from build123d import *

# Parameters (mm, degrees)
F0_W     = 31
F0_H     = 13
F1_DEPTH = 2
F2_R     = 1.55
F3_DEPTH = 25
F4_R     = 2
F5_W     = 15
F5_H     = 5
F6_DEPTH = 25
F7_R     = 1
F8_R     = 0.2


with BuildPart() as f1:
    # F0 (on Front) → F1 (new body)
    with BuildSketch(Plane.XZ):
        with Locations((15.5, 6.5)):
            Rectangle(F0_W, F0_H)
    extrude(amount=F1_DEPTH)

    # F2 (on face) → F3 (cut)
    with BuildSketch(Plane.XZ.offset(2)):
        with Locations((4, 10)):
            Circle(F2_R)
        with Locations((4, 3)):
            Circle(F2_R)
        with Locations((27, 10)):
            Circle(F2_R)
        with Locations((27, 3)):
            Circle(F2_R)
    extrude(amount=-F3_DEPTH, mode=Mode.SUBTRACT)

    # F4
    f4_edges = [f1.edges().sort_by_distance(p)[0] for p in [
        (31, -1, 13),
        (31, -1, 0),
        (0, -1, 0),
        (0, -1, 13),
    ]]
    fillet(f4_edges, radius=F4_R)

    # F5 (on face) → F6 (cut)
    with BuildSketch(Plane.XZ.offset(2)):
        with Locations((15.5, 6.5)):
            Rectangle(F5_W, F5_H)
    extrude(amount=-F6_DEPTH, mode=Mode.SUBTRACT)

    # F7
    f7_edges = [f1.edges().sort_by_distance(p)[0] for p in [
        (8, -1, 9),
        (8, -1, 4),
        (23, -1, 9),
        (23, -1, 4),
    ]]
    fillet(f7_edges, radius=F7_R)

    # F8
    f8_edges = [f1.edges().sort_by_distance(p)[0] for p in [
        (15.5, -2, 9),
        (22.707107, -2, 8.707107),
        (23, -2, 6.5),
        (22.707107, -2, 4.292893),
        (15.5, -2, 4),
        (8.292893, -2, 4.292893),
        (8, -2, 6.5),
        (8.292893, -2, 8.707107),
    ]]
    fillet(f8_edges, radius=F8_R)


solid = f1.part
Work out the finished part from the listing and answer in its coordinate system (mm). A direction names the side the tool comes from. Round coordinates to 2 decimals unless told otherwise and drop trailing zeros. Write each loop counter-clockwise with the first axis right and the second up, starting at its lowest first coordinate (ties: lowest second). Pieces come first, ordered by that corner, then holes. Notation, with made-up numbers: (49.25, 60.25) -> (54.25, 60.25) arc R13 cw to (54.25, 73.25) -> close; hole circle Ø4 at (82.25, 9.5). An arc over 180 degrees is marked (long way). Answer as CSV lines item,"result". Start each with the question number.
(1) The part is cut by section B-B, the plane x = 27. Give the vertices of the cut face in (y, z), then the cut area to 3 significant figures.
(2) A tool of negligible diameter and unlimited length cuts with its end or side. For faces 1 (the flat face through (15, -1, 9)), 2 (the flat face through (15, -1, 13)), from which of +Z, -Z, +X, -X, +Y, -Y can it reach the whole face along a straight path? Write none if from no direction.
(3) The part is cut by section C-C, the plane y = -1.1. Give the vertices of the cut face in (x, z), then the cut area to 3 significant figures.
(4) The mould has two halves that part along Z. Classify faces 3 (the cylindrical face through (22.699, -0.887, 4.285)), 4 (the cylindrical face through (30.4, -1.01, 0.57)), 5 (the cylindrical face through (30.4, -1.01, 12.43)), 6 (the cylindrical face through (2.77, -1.01, 2.06)): +Z half, -Z half, draft (parallel to the pull), parting line (faces both ways), or undercut.
(5) The part is cut by section D-D, the plane x = 20. Give the vertices of the cut face in (y, z), then the cut area to 3 significant figures.
(6) Find the intervals of material crossed by probe 1 along Z at (x, y) = (4, -0.5); probe 2 along Z at (x, y) = (21, -0.3); probe 3 along X at (y, z) = (-0.6, 6.25), in increasing order.
(7) The part is cut by section A-A, the plane z = 3. Give the vertices of the cut face in (x, y), then the cut area to 3 significant figures.
Output values:
1,outline,"(-2, 0) -> (0, 0) -> (0, 1.45) -> (-2, 1.45) -> close; (-2, 4.55) -> (0, 4.55) -> (0, 8.45) -> (-2, 8.45) -> close; (-2, 11.55) -> (0, 11.55) -> (0, 13) -> (-2, 13) -> close"
1,area,"13.6 mm²"
2,face 1,"+Y, -Y"
2,face 2,"+Z, +X, -X, +Y, -Y"
3,outline,"(0, 2) arc R2 ccw to (2, 0) -> (29, 0) arc R2 ccw to (31, 2) -> (31, 11) arc R2 ccw to (29, 13) -> (2, 13) arc R2 ccw to (0, 11) -> close; hole circle Ø3.1 at (4, 3); hole circle Ø3.1 at (4, 10); hole (8, 5) arc R1 ccw to (9, 4) -> (22, 4) arc R1 ccw to (23, 5) -> (23, 8) arc R1 ccw to (22, 9) -> (9, 9) arc R1 ccw to (8, 8) -> close; hole circle Ø3.1 at (27, 3); hole circle Ø3.1 at (27, 10)"
3,area,"295 mm²"
4,face 3,"undercut"
4,face 4,"-Z half"
4,face 5,"+Z half"
4,face 6,"undercut"
5,outline,"(-2, 0) -> (0, 0) -> (0, 4) -> (-1.8, 4) arc R0.2 ccw to (-2, 3.8) -> close; (-2, 9.2) arc R0.2 ccw to (-1.8, 9) -> (0, 9) -> (0, 13) -> (-2, 13) -> close"
5,area,"16.0 mm²"
6,probe 1,"z = 0 to 1.45, 4.55 to 8.45, 11.55 to 13"
6,probe 2,"z = 0 to 4, 9 to 13"
6,probe 3,"x = 0 to 8, 23 to 31"
7,outline,"(0, -2) -> (2.45, -2) -> (2.45, 0) -> (0, 0) -> close; (5.55, -2) -> (25.45, -2) -> (25.45, 0) -> (5.55, 0) -> close; (28.55, -2) -> (31, -2) -> (31, 0) -> (28.55, 0) -> close"
7,area,"49.6 mm²"
